The model under review builds one solid part; all positions refer to its coordinate system, in mm. A direction names the side the tool comes from. Round coordinates to 2 decimals unless told otherwise and drop trailing zeros. Loops run counter-clockwise (first coordinate to the right, second up) from the corner with the lowest first, then second, coordinate; pieces in that order, holes last. Notation, with made-up numbers: M 26.25,11.25 L 54.25,11.25 A17 ccw 54.25,29.25 Z; hole C -35.75,-26.5 d7. An arc over 180 degrees is marked long. Answer as a JSON object with one key per item and string values. Group by question number.
Item 1: Consider section B-B (y = -16.25). Give the boundary of the cut face in (x, z).
Item 2: Consider section D-D (x = -13). Give the boundary of the cut face in (y, z), and give its area (3 significant figures).
Item 3: Tool access review of faces 5 (the face through (-40.3, -12.5, 40)), 6 (the face through (2.816, -13, -4)): name each direction out of +Z, -Z, +X, -X, +Y, -Y from which nothing blocks a thin tool from reaching the whole face with its end or side.
Item 4: Consider section C-C (z = -5.5). Give the boundary of the cut face in (x, y).
Item 5: The part is to be moulded in two halves that separate along Z. For faces 1 (the face through (-40, 0, -4)), 2 (the face through (7.355, -12.522, 39.91)), 3 (the face through (-16, -13, 38.191)), 4 (the face through (-16, -13, 39.337)), say which applies: +Z half, -Z half, draft (parallel to the pull), parting line (faces both ways), or undercut.
Item 6: Consider section A-A (x = -5.5). Give the boundary of the cut face in (y, z), and give its area (3 significant figures).
Item 7: To check wall thickness, follow line 1 (Z direction, x = -11, y = -9); line 2 (Z direction, x = -31, y = -14.25); line 3 (X direction, y = -1.5, z = -8). State the ranges of each line that lie inside material, in increasing order.
Item 8: Insertion check: P1, Ø1.5, axis at x = -33.5, y = -19, coming from the -Z side; P2, Ø0.6, axis at y = -16, z = 38.5, coming from the -X side. Each pin has a flat end and moves straight along its axis. Give the tip position at first contact, or say it passes through.
```python
from build123d import *

# Parameters (mm, degrees)
F0_W     = 10.8844153583
F0_H     = 1.1457279325
F1_DEPTH = 25.4


with BuildPart() as f1:
    # F0 (on Front) → F1 (new body)
    with BuildSketch(Plane.XZ):
        with BuildLine():
            Line((2.8158243909, 41.8190695345), (-35.8509788454, 41.8190695345))
            ThreePointArc((-35.8509788454, 41.8190695345), (-40.3411069059, 39.9591975951), (-42.2009788454, 35.4690695345))
            Line((-42.2009788454, 35.4690695345), (-42.2009788454, -44.8258476496))
            ThreePointArc((-42.2009788454, -44.8258476496), (-40.3411069059, -49.3159757101), (-35.8509788454, -51.1758476496))
            Line((-35.8509788454, -51.1758476496), (-16.8040137117, -51.1758476496))
            ThreePointArc((-16.8040137117, -51.1758476496), (-19.7564134277, -48.2901591682), (-17.5108828007, -44.8258476496))
            Line((-17.5108828007, -44.8258476496), (-35.8509788454, -44.8258476496))
            Line((-35.8509788454, -44.8258476496), (-35.8509788454, 35.4690695345))
            Line((-35.8509788454, 35.4690695345), (2.8158243909, 35.4690695345))
            Line((2.8158243909, 35.4690695345), (2.8158243909, -44.8258476496))
            Line((2.8158243909, -44.8258476496), (-15.5242716537, -44.8258476496))
            ThreePointArc((-15.5242716537, -44.8258476496), (-13.8853656886, -46.0082877402), (-13.2587354849, -47.9296185076))
            ThreePointArc((-13.2587354849, -47.9296185076), (-14.114090107, -50.1303681901), (-16.2311407427, -51.1758476496))
            Line((-16.2311407427, -51.1758476496), (2.8158243909, -51.1758476496))
            ThreePointArc((2.8158243909, -51.1758476496), (7.3059524515, -49.3159757101), (9.1658243909, -44.8258476496))
            Line((9.1658243909, -44.8258476496), (9.1658243909, 35.4690695345))
            ThreePointArc((9.1658243909, 35.4690695345), (7.3059524515, 39.9591975951), (2.8158243909, 41.8190695345))
        make_face()
        with Locations((-16.135668382, 38.763795048)):
            Rectangle(F0_W, F0_H, mode=Mode.SUBTRACT)
        with BuildLine():
            ThreePointArc((-17.5108828007, -44.8258476496), (-19.7564134277, -48.2901591682), (-16.8040137117, -51.1758476496))
            Line((-16.8040137117, -51.1758476496), (-16.2311407427, -51.1758476496))
            ThreePointArc((-16.2311407427, -51.1758476496), (-14.114090107, -50.1303681901), (-13.2587354849, -47.9296185076))
            ThreePointArc((-13.2587354849, -47.9296185076), (-13.8853656886, -46.0082877402), (-15.5242716537, -44.8258476496))
            Line((-15.5242716537, -44.8258476496), (-17.5108828007, -44.8258476496))
        make_face()
        with BuildLine():
            Line((-16.2311407427, -51.1758476496), (-16.8040137117, -51.1758476496))
            ThreePointArc((-16.8040137117, -51.1758476496), (-16.5175772272, -51.18846025), (-16.2311407427, -51.1758476496))
        make_face()
    extrude(amount=F1_DEPTH)


solid = f1.part
```
Geometry results:
{
 "1": {"outline": "M -42.2,-44.83 A6.35 ccw -35.85,-51.18 L -16.8,-51.18 A3.26 ccw -16.23,-51.18 L 2.82,-51.18 A6.35 ccw 9.17,-44.83 L 9.17,35.47 A6.35 ccw 2.82,41.82 L -35.85,41.82 A6.35 ccw -42.2,35.47 Z; hole M -35.85,-44.83 L 2.82,-44.83 L 2.82,35.47 L -35.85,35.47 Z; hole M -21.58,38.19 L -10.69,38.19 L -10.69,39.34 L -21.58,39.34 Z"},
 "2": {"outline": "M -25.4,-51.18 L 0,-51.18 L 0,-44.83 L -25.4,-44.83 Z; M -25.4,35.47 L 0,35.47 L 0,38.19 L -25.4,38.19 Z; M -25.4,39.34 L 0,39.34 L 0,41.82 L -25.4,41.82 Z", "area": "293 mm^2"},
 "3": {"face 5": "+Z, -X, +Y, -Y", "face 6": "+Y, -Y"},
 "4": {"outline": "M -42.2,-25.4 L -35.85,-25.4 L -35.85,0 L -42.2,0 Z; M 2.82,-25.4 L 9.17,-25.4 L 9.17,0 L 2.82,0 Z"},
 "5": {"face 1": "draft", "face 2": "+Z half", "face 3": "undercut", "face 4": "undercut"},
 "6": {"outline": "M -25.4,-51.18 L 0,-51.18 L 0,-44.83 L -25.4,-44.83 Z; M -25.4,35.47 L 0,35.47 L 0,41.82 L -25.4,41.82 Z", "area": "323 mm^2"},
 "7": {"line 1": "z = -51.18 to -44.83, 35.47 to 38.19, 39.34 to 41.82", "line 2": "z = -51.18 to -44.83, 35.47 to 41.82", "line 3": "x = -42.2 to -35.85, 2.82 to 9.17"},
 "8": {"P1": "stops at z = -51.18", "P2": "stops at x = -41.58"}
}
